Job drawing, mm, ordinate dimensions from the low corner. One solid piece. Round coordinates to 2 decimals unless told otherwise and drop trailing zeros. Loops run counter-clockwise (first coordinate to the right, second up) from the corner with the lowest first, then second, coordinate; pieces in that order, holes last. Notation, with made-up numbers: M 48,-33 L 86,-33 A34 ccw 86,5 Z; hole C 65.5,-33 d9. An arc over 180 degrees is marked long. Use a Markdown table: item, result. Add a question column.
(1) Flat gauge pin, fed straight in: P1, Ø14, axis at x = 14.29, z = 15.33, coming from the +Y side. Where does the tip first touch, or does it go through?
(2) Band-saw the part on A-A, the plane x = 14.29. Write the cut outline in (y, z), and give its area (3 significant figures).
(3) Band-saw the part on B-B, the plane z = 15.33. Write the cut outline in (x, y), and give its area (3 significant figures).
(4) Band-saw the part on D-D, the plane x = 5.25. Write the cut outline in (y, z).
(5) Band-saw the part on C-C, the plane y = 8. Write the cut outline in (x, z), and give its area (3 significant figures).
(6) Wall check: L1, parallel to X at y = 4.5, z = 15.33; L2, parallel to Z at x = 11.5, y = 7; L3, parallel to Z at x = 8.75, y = 10.25. Give the ranges that are in metal, low to high.
(7) Two-plate mould, pull along X, no slides. Class the marked faces 1, 2, 3 and 4: released by +X, released by -X, zero draft, split by the parting line, or undercut.
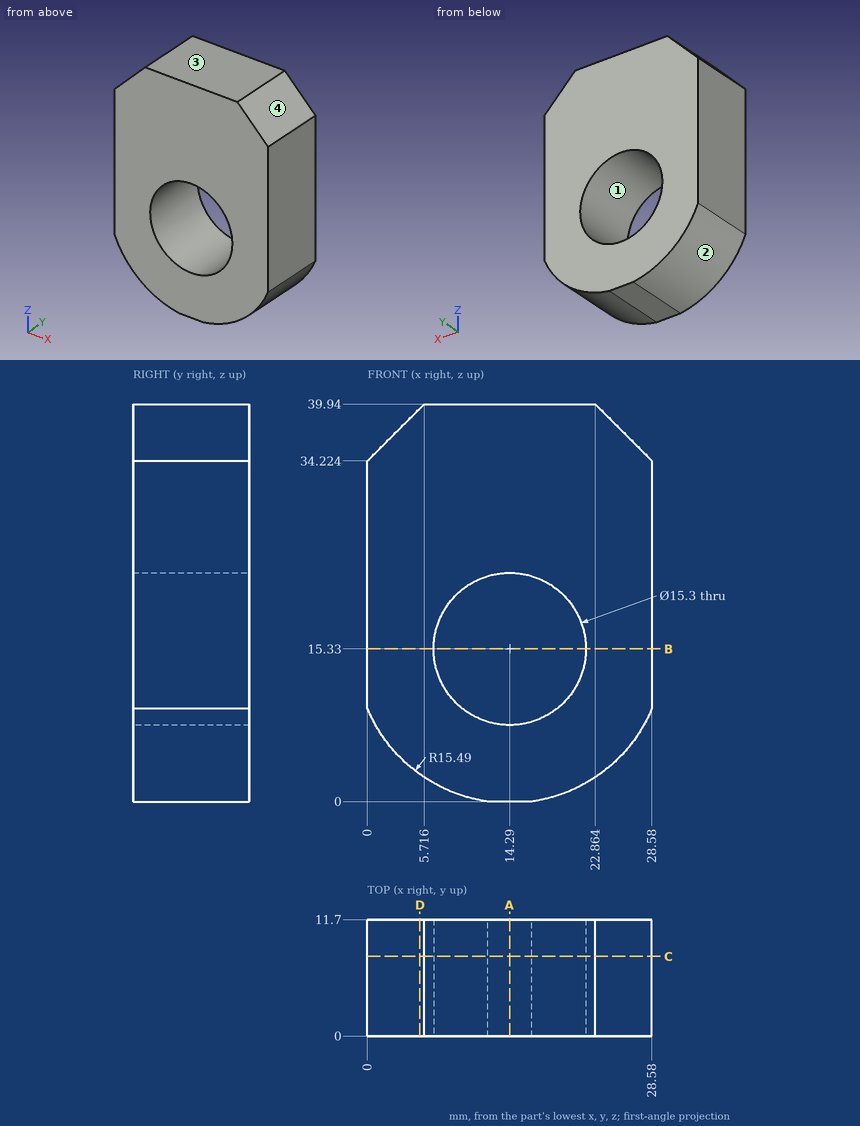
Return value:
| question | item | result |
|---|---|---|
| 1 | P1 | through |
| 2 | outline | M 0,0 L 11.7,0 L 11.7,7.68 L 0,7.68 Z; M 0,22.98 L 11.7,22.98 L 11.7,39.94 L 0,39.94 Z |
| 2 | area | 288 mm^2 |
| 3 | outline | M 0,0 L 6.64,0 L 6.64,11.7 L 0,11.7 Z; M 21.94,0 L 28.58,0 L 28.58,11.7 L 21.94,11.7 Z |
| 3 | area | 155 mm^2 |
| 4 | outline | M 0,2.75 L 11.7,2.75 L 11.7,39.47 L 0,39.47 Z |
| 5 | outline | M 0,9.35 A15.49 ccw 12.07,0 L 16.51,0 A15.49 ccw 28.58,9.35 L 28.58,34.22 L 22.86,39.94 L 5.72,39.94 L 0,34.22 Z; hole C 14.29,15.33 d15.3 |
| 5 | area | 854 mm^2 |
| 6 | L1 | 0 to 6.64, 21.94 to 28.58 |
| 6 | L2 | 0.09 to 8.21, 22.45 to 39.94 |
| 6 | L3 | 0.86 to 10.05, 20.61 to 39.94 |
| 7 | face 1 | undercut |
| 7 | face 2 | released by -X |
| 7 | face 3 | zero draft |
| 7 | face 4 | released by +X |
